Here's how the part is built. I have some questions about the finished solid (model axes, mm). Round coordinates to 2 decimals unless told otherwise and drop trailing zeros. Write each loop counter-clockwise with the first axis right and the second up, starting at its lowest first coordinate (ties: lowest second). Pieces come first, ordered by that corner, then holes. Notation, with made-up numbers: (72.5, 80.5) - (107.5, 80.5) arc R12 ccw to (107.5, 90.5) - close; hole circle Ø5 at (71, 81.25). An arc over 180 degrees is marked (long way). Write item = value, one per line. Start each with the question number.
Item 1: If I drill on line 1 along Z through (x, y) = (-16, 6.75); line 2 along Z through (x, y) = (-16.25, 1.5); line 3 along Y through (x, z) = (-17.5, -100.5), over which ranges is the centre line in solid material (lowest first)? Write a range as [from, to].
Item 2: Thinking about a two-plate mould opening in Z: for faces 1 (the face through (-18, 4, -107.5)), 2 (the face through (-17.59, 5.66, -7.37)), 3 (the face through (-18, 4, 0)), 4 (the face through (-19, 8, -53)), which applies, pulls with the +Z half, pulls with the -Z half, needs draft (parallel to the pull), parting line crosses it, or undercut?
Item 3: If we section it at B-B (z = -7): Please give me the cut outline in (x, y), and give its area (3 significant figures).
Item 4: For P1, Ø2.5, axis at y = 4, z = -100.5, coming from the +X side, with a flat end and sliding along its axis, tell me the tip position at first contact or that it passes through.
Item 5: If we section it at A-A (y = 4): Give the number of separate pieces and of enclosed holes in the cut face, and give its area (3 significant figures).
Autodesk Inventor part; units mm, degrees
ref_plane "YZ Plane" through (0, 0, 0) normal (1, 0, 0) x (0, 1, 0)
ref_plane "XZ Plane" through (0, 0, 0) normal (0, 1, 0) x (-1, 0, 0)
ref_plane "XY Plane" through (0, 0, 0) normal (0, 0, 1) x (1, 0, 0)
sketch "Sketch1" plane through (0, 0, 0) normal (0, 1, 0) x (-1, 0, 0)
  line L0 (0, 0) -> (11.75, 0)
  line L1 (11.75, 0) -> (11.75, -102.5)
  line L2 (10.25, -107.5) -> (0, -107.5)
  line L3 (0, -107.5) -> (0, 0)
  circle A0 centre (11.75, -23.75) radius 8.75
  circle A1 centre (11.75, -43.75) radius 8.75
  circle A2 centre (11.75, -63.75) radius 8.75
  circle A3 centre (11.75, -83.75) radius 8.75
  line L4 (11.75, 0) -> (23.5, 0)
  line L5 (23.5, 0) -> (23.5, -107.5)
  line L6 (23.5, -107.5) -> (13.25, -107.5)
  line L7 (13.25, -107.5) -> (13.25, -92.3705)
  line L8 (13.25, -75.1295) -> (13.25, -72.3705)
  line L9 (13.25, -55.1295) -> (13.25, -52.3705)
  line L10 (13.25, -32.3705) -> (13.25, -35.1295)
  line L11 (13.25, -15.1295) -> (13.25, 0)
  line L12 (10.25, 0) -> (10.25, -15.1295)
  line L13 (10.25, -32.3705) -> (10.25, -35.1295)
  line L14 (10.25, -52.3705) -> (10.25, -55.1295)
  line L15 (10.25, -72.3705) -> (10.25, -75.1295)
  line L16 (10.25, -92.3705) -> (10.25, -107.5)
  point P0 (11.75, -92.5)
  point P1 (11.75, -75)
  point P2 (11.75, -72.5)
  point P3 (11.75, -55)
  point P4 (11.75, -52.5)
  point P5 (11.75, -35)
  point P6 (11.75, -32.5)
  point P7 (11.75, -15)
  dimension "d0" = 17.5
  dimension "d4" = 20
  dimension "d9" = 3
  dimension "d11" = 15
  dimension "d12" = 15
  dimension "d16" = 1.5
  dimension "d17" = 3
  dimension "d19" = 1.5
extrude "Extrusion1" add sketch "Sketch1" along normal blind 8 contours L4 L5 L6 L7 A3 L8 A2 L9 A1 L10 A0 L11
sketch "Sketch3" plane through (-23.5, 0, -107.5) normal (-1, 0, 0) x (0, 0, 1)
  line L0 (0, 0) -> (0, 8)
  line L1 (0, 8) -> (107.5, 8)
  line L2 (107.5, 0) -> (107.5, 8)
  point P0 (7, 4)
  point P1 (100.5, 4)
  point P2 (107.5, 4)
  dimension "d27" = 7
  dimension "d28" = 8
  dimension "d29" = 4
  dimension "d33" = 7
hole "Hole1" at (-23.5, 4, -100.5) at (-23.5, 4, -7) direction (1, 0, 0) diameter 3.4 end through all countersink diameter 6.3 countersink angle 90
fillet "Fillet1" radius 1 8 edges at (-13.25, 4, -92.3705) (-13.25, 4, -72.3705) (-13.25, 4, -75.1295) (-13.25, 4, -55.1295) (-13.25, 4, -52.3705) (-13.25, 4, -35.1295) (-13.25, 4, -32.3705) (-13.25, 4, -15.1295)
chamfer "Chamfer1" distance 0.5 angle 45 40 edges at (-20.5, 0, -83.75) (-13.4574, 0, -92.5643) (-13.25, 0, -100.337) (-13.4574, 0, -74.9357) (-13.25, 0, -73.75) (-13.4574, 0, -72.5643) (-20.5, 0, -63.75) (-13.4574, 0, -54.9357) (-13.25, 0, -53.75) (-13.4574, 0, -52.5643) (-20.5, 0, -43.75) (-13.4574, 0, -34.9357) (-13.25, 0, -33.75) (-13.4574, 0, -32.5643) (-20.5, 0, -23.75) (-13.4574, 0, -14.9357) (-13.25, 0, -7.163) (-23.5, 0, -53.75) (-18.375, 0, -107.5) (-18.375, 0, 0) (-23.5, 8, -53.75) (-20.5, 8, -23.75) (-13.4574, 8, -32.5643) (-13.25, 8, -33.75) (-13.4574, 8, -34.9357) (-20.5, 8, -43.75) (-13.4574, 8, -52.5643) (-13.25, 8, -53.75) (-13.4574, 8, -54.9357) (-20.5, 8, -63.75) (-13.4574, 8, -72.5643) (-13.25, 8, -73.75) (-13.4574, 8, -74.9357) (-20.5, 8, -83.75) (-13.4574, 8, -92.5643) (-13.25, 8, -100.337) (-13.4574, 8, -14.9357) (-13.25, 8, -7.163) (-18.375, 8, -107.5) (-18.375, 8, 0)
equation "\"d12\" = d11"
equation "\"d19\" = d16"
properties part number "BatteryHolder" material "Aluminum 6061"
Reply:
q1.line_1 = [-107.5, -91.4], [-76.1, -71.4], [-56.1, -51.4], [-36.1, -31.4], [-16.1, 0]
q1.line_2 = [-107.5, -91.25], [-76.25, -71.25], [-56.25, -51.25], [-36.25, -31.25], [-16.25, 0]
q1.line_3 = [0, 2.3], [5.7, 8]
q2.face_1 = pulls with the -Z half
q2.face_2 = undercut
q2.face_3 = pulls with the +Z half
q2.face_4 = needs draft
q3.outline = (-23.5, 0.5) - (-23, 0) - (-13.75, 0) - (-13.25, 0.5) - (-13.25, 2.3) - (-22.05, 2.3) - (-23.5, 0.85) - close; (-23.5, 7.15) - (-22.05, 5.7) - (-13.25, 5.7) - (-13.25, 7.5) - (-13.75, 8) - (-23, 8) - (-23.5, 7.5) - close
q3.area = 44.5 mm2
q4.P1 = through
q5.separate_pieces = 3
q5.enclosed_holes = 0
q5.area = 650 mm2
